Verification items for the finished model (mm, model axes). Face numbers are marked on the shaded views. Round coordinates to 2 decimals unless told otherwise and drop trailing zeros. Order: outer loops, then holes, each group sorted by start corner. A loop starts at its lowest first (then second) coordinate and runs counter-clockwise, first axis right, second up. Notation, with made-up numbers: (63, 54.25) -> (76, 54.25) arc R18 cw to (76, 86.25) -> close; hole circle Ø6 at (40.5, -22.5). An arc over 180 degrees is marked (long way). Return JSON: item names as keys, results as strings. Group by question number.
Item 1: Sectioned sample at A-A on z = -5.5. Record the cut outline in (x, y), plus the area to 3 significant figures.
Item 2: Sectioned sample at C-C on x = 5.35. Record the cut outline in (y, z), plus the area to 3 significant figures.
Item 3: Sectioned sample at D-D on z = 4.85. Record the cut outline in (x, y).
Item 4: Draft check along Z on the marked faces 1, 2, 3 and 4. Enter one of: pulls with the +Z half, pulls with the -Z half, needs draft (parallel to the pull), parting line crosses it, or undercut.
Item 5: Sectioned sample at B-B on y = -0.4. Record the cut outline in (x, z).
Item 6: Scan lines: probe 1 along X at (y, z) = (-0.75, -4.85); probe 2 along Z at (x, y) = (5.5, -1.1); probe 3 along Z at (x, y) = (5, -0.45). Record each from-to range of solid material in increasing order. Write a range as from..to.
Item 7: Depth check by flat-ended pin: pin 1 Ø2 at (x, z) = (-8.5, 3) entering from +Y; pin 2 Ø2 at (x, z) = (5.35, -4.85) entering from -Y. Enter the tip coordinate at first touch or a pass-through.
```python
from build123d import *

# Parameters (mm, degrees)
SKETCH1_R           = 1.25
BOSS_EXTRUDE1_DEPTH = 1.6


with BuildPart() as part:
    # Sketch1 → Boss-Extrude1 (new body)
    with BuildSketch(Plane(origin=(0, 0, 0), x_dir=(1, 0, 0), z_dir=(0, 1, 0))):
        with BuildLine():
            Line((-11.1, 7), (4.75, 7))
            ThreePointArc((4.75, 7), (6.871320344, 6.121320344), (7.75, 4))
            Line((7.75, 4), (7.75, -4))
            ThreePointArc((7.75, -4), (6.871320344, -6.121320344), (4.75, -7))
            Line((4.75, -7), (-11.1, -7))
            ThreePointArc((-11.1, -7), (-13.221320344, -6.121320344), (-14.1, -4))
            Line((-14.1, -4), (-14.1, 4))
            ThreePointArc((-14.1, 4), (-13.221320344, 6.121320344), (-11.1, 7))
        make_face()
        with Locations(Location((5.35, 4.85, 0), (0, 0, 270))):
            Circle(SKETCH1_R, mode=Mode.SUBTRACT)
        with Locations(Location((5.35, -4.85, 0), (0, 0, 270))):
            Circle(SKETCH1_R, mode=Mode.SUBTRACT)
    extrude(amount=-BOSS_EXTRUDE1_DEPTH)


solid = part.part
```
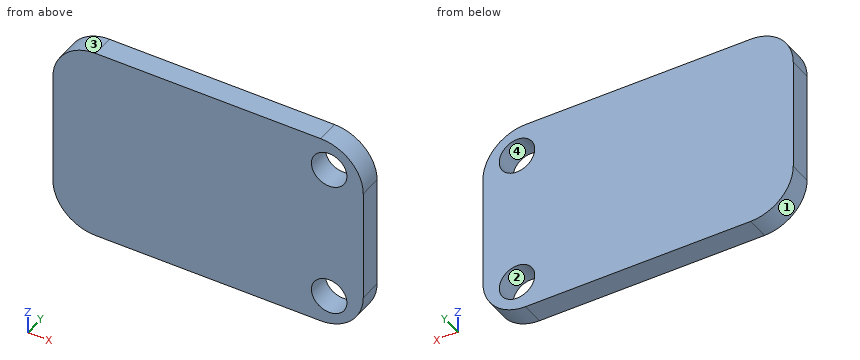
Recorded:
{
 "1": {"outline": "(-13.7, -1.6) -> (4.28, -1.6) -> (4.28, 0) -> (-13.7, 0) -> close; (6.42, -1.6) -> (7.35, -1.6) -> (7.35, 0) -> (6.42, 0) -> close", "area": "30.3 mm²"},
 "2": {"outline": "(-1.6, -6.94) -> (0, -6.94) -> (0, -6.1) -> (-1.6, -6.1) -> close; (-1.6, -3.6) -> (0, -3.6) -> (0, 3.6) -> (-1.6, 3.6) -> close; (-1.6, 6.1) -> (0, 6.1) -> (0, 6.94) -> (-1.6, 6.94) -> close", "area": "14.2 mm²"},
 "3": {"outline": "(-13.98, -1.6) -> (4.1, -1.6) -> (4.1, 0) -> (-13.98, 0) -> close; (6.6, -1.6) -> (7.63, -1.6) -> (7.63, 0) -> (6.6, 0) -> close"},
 "4": {"face 1": "pulls with the -Z half", "face 2": "undercut", "face 3": "pulls with the +Z half", "face 4": "undercut"},
 "5": {"outline": "(-14.1, -4) arc R3 ccw to (-11.1, -7) -> (4.75, -7) arc R3 ccw to (7.75, -4) -> (7.75, 4) arc R3 ccw to (4.75, 7) -> (-11.1, 7) arc R3 ccw to (-14.1, 4) -> close; hole circle Ø2.5 at (5.35, -4.85); hole circle Ø2.5 at (5.35, 4.85)"},
 "6": {"probe 1": "-13.98..4.1, 6.6..7.63", "probe 2": "-6.9..-6.09, -3.61..3.61, 6.09..6.9", "probe 3": "-6.99..-6.05, -3.65..3.65, 6.05..6.99"},
 "7": {"pin 1": "y = 0", "pin 2": "through"}
}
